Autodesk Inventor part; units mm, degrees
ref_plane "YZ Plane" through (0, 0, 0) normal (1, 0, 0) x (0, 1, 0)
ref_plane "XZ Plane" through (0, 0, 0) normal (0, 1, 0) x (-1, 0, 0)
ref_plane "XY Plane" through (0, 0, 0) normal (0, 0, 1) x (1, 0, 0)
sketch "Sketch1" plane through (0, 0, 0) normal (0, 0, 1) x (1, 0, 0)
  line L0 (-35, 40) -> (35, 40)
  line L1 (40, 35) -> (40, -35)
  line L2 (35, -40) -> (-35, -40)
  line L3 (-40, -35) -> (-40, 35)
  line L4 (-40, 40) -> (40, -40) construction
  line L5 (40, 40) -> (-40, -40) construction
  arc A0 (-35, 40) -> (-40, 35) centre (-35, 35) ccw
  arc A1 (40, 35) -> (35, 40) centre (35, 35) ccw
  arc A2 (35, -40) -> (40, -35) centre (35, -35) ccw
  arc A3 (-40, -35) -> (-35, -40) centre (-35, -35) ccw
  line L6 (35, 38) -> (-35, 38)
  arc A4 (-35, 38) -> (-38, 35) centre (-35, 35) ccw
  line L7 (-38, 35) -> (-38, -35)
  arc A5 (-38, -35) -> (-35, -38) centre (-35, -35) ccw
  line L8 (-35, -38) -> (35, -38)
  arc A6 (35, -38) -> (38, -35) centre (35, -35) ccw
  line L9 (38, -35) -> (38, 35)
  arc A7 (38, 35) -> (35, 38) centre (35, 35) ccw
  point P0 (0, 0)
  dimension "d0" = 80
  dimension "d1" = 5
  dimension "d2" = 2
extrude "Extrusion1" add sketch "Sketch1" along normal blind 320
sketch "Sketch2" plane through (0, 0, 0) normal (0, 1, 0) x (-1, 0, 0)
  line L0 (40, 0) -> (40, 320)
  line L1 (-40, 0) -> (-40, 320)
  line L2 (40, 320) -> (-40, 320)
  line L3 (40, 320) -> (-40, 200.9923)
  point P0 (0, 0)
  dimension "d5" = 123.91
extrude "Extrusion2" cut sketch "Sketch2" along normal through all both and the other way through all
properties part number "MSC 903 base tube"
Verification items for the finished model (mm, model axes). A direction names the side the tool comes from. Coordinates: 2 decimals unless noted, no trailing zeros. Loops run counter-clockwise (first coordinate to the right, second up) from the corner with the lowest first, then second, coordinate; pieces in that order, holes last. Notation, with made-up numbers: (22, 72) -> (62, 72) arc R27 ccw to (62, 91) -> close; hole circle Ø6 at (77, -4). An arc over 180 degrees is marked (long way). Answer as a JSON object with one key per item and string values. Group by question number.
Item 1: Tool access check on faces 1 (the flat face through (38, 0, 101)), 2 (the flat face through (40, 0, 99)). Record the directions out of +Z, -Z, +X, -X, +Y, -Y that give a thin tool (end or side, any length) a straight path to the whole face; none if there is none.
Item 2: Mould release check, pull along X, two halves, no side actions. Record for faces 3 (the flat face through (-0.2, -38.3, 0)), 4 (the flat face through (-40, 0, 158)), 5 (the flat face through (0, -38, 119)): +X half, -X half, draft (parallel to the pull), parting line (faces both ways), or undercut.
Item 3: Sectioned sample at D-D on z = 213. Record the boundary of the cut face in (x, y), plus the area to 3 significant figures.
Item 4: Scan lines: probe 1 along X at (y, z) = (26, 30); probe 2 along X at (y, z) = (30.5, 307). Record each from-to range of solid material in increasing order.
Item 5: Sectioned sample at B-B on x = 29. Record the boundary of the cut face in (y, z), plus the area to 3 significant figures.
Item 6: Sectioned sample at C-C on z = 32. Record the boundary of the cut face in (x, y).
Item 7: Sectioned sample at A-A on y = -13. Record the boundary of the cut face in (x, z), plus the area to 3 significant figures.
Evaluation:
{
 "1": {"face 1": "+Z, -Z", "face 2": "+Z, -Z, +X, +Y, -Y"},
 "2": {"face 3": "draft", "face 4": "-X half", "face 5": "undercut"},
 "3": {"outline": "(-40, -35) arc R5 ccw to (-35, -40) -> (31.93, -40) -> (31.93, -38) -> (-35, -38) arc R3 cw to (-38, -35) -> (-38, 35) arc R3 cw to (-35, 38) -> (31.93, 38) -> (31.93, 40) -> (-35, 40) arc R5 ccw to (-40, 35) -> close", "area": "433 mm²"},
 "4": {"probe 1": "x = -40 to -38, 38 to 40", "probe 2": "x = -40 to -38"},
 "5": {"outline": "(-40, 0) -> (-38, 0) -> (-38, 217.36) -> (-40, 217.36) -> close; (38, 0) -> (40, 0) -> (40, 217.36) -> (38, 217.36) -> close", "area": "869 mm²"},
 "6": {"outline": "(-40, -35) arc R5 ccw to (-35, -40) -> (35, -40) arc R5 ccw to (40, -35) -> (40, 35) arc R5 ccw to (35, 40) -> (-35, 40) arc R5 ccw to (-40, 35) -> close; hole (-38, -35) arc R3 ccw to (-35, -38) -> (35, -38) arc R3 ccw to (38, -35) -> (38, 35) arc R3 ccw to (35, 38) -> (-35, 38) arc R3 ccw to (-38, 35) -> close"},
 "7": {"outline": "(-40, 0) -> (-38, 0) -> (-38, 317.02) -> (-40, 320) -> close; (38, 0) -> (40, 0) -> (40, 200.99) -> (38, 203.97) -> close", "area": "1,040 mm²"}
}
